Verification items for the finished model (mm, model axes). Coordinates: 2 decimals unless noted, no trailing zeros.
Q1. Cross-section at A-A, the plane y = 1.35. Count the separate pieces of the cut face and the enclosed holes in it, and give its area (3 significant figures).
Q2. Thickness scan on line 1 (X direction, y = 2.6, z = 25) (3 decimals); line 2 (Z direction, x = -38, y = 1.25); line 3 (Z direction, x = 1.5, y = 1.35). Record the ranges inside material, lowest first.
Q3. Depth check by flat-ended pin: P1, Ø5, axis at x = -38.1, z = -66.675, coming from the +Y side (3 decimals); P2, Ø2.5, axis at x = 14.22, z = 83.02, coming from the +Y side. Enter the tip coordinate at first touch or a pass-through.
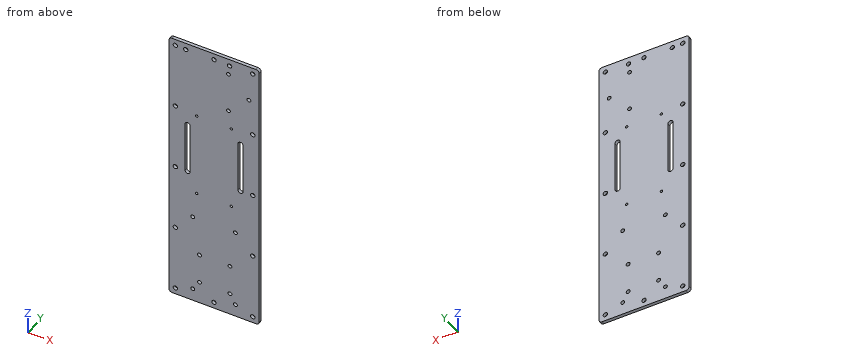
from build123d import *

# Parameters (mm, degrees)
PLATE_THICKNESS_DEPTH      = 3.175
SKETCH3_R                  = 2.159
MOUNTING_HOLES_DEPTH       = 147.635511132
SKETCH4_R                  = 1.905
JETSON_HOLES_W_MOUNT_DEPTH = 147.635511132
SKETCH5_R                  = 1.905
PDB_HOLES_DEPTH            = 147.635511132
SKETCH6_R                  = 1.905
LIDAR_HOLES_DEPTH          = 147.635511132
SKETCH7_R                  = 1.27
PIXHAWK_HOLES_DEPTH        = 147.635511132
BATTERY_HOLES_DEPTH        = 147.635511132
SKETCH9_R                  = 2.159
CUT_EXTRUDE1_DEPTH         = 147.635511132


with BuildPart() as part:
    # Sketch2 → Plate Thickness (new body)
    with BuildSketch(Plane(origin=(0, 0, 0), x_dir=(1, 0, 0), z_dir=(0, 1, 0))):
        with BuildLine():
            Line((-41.275, 139.7), (41.275, 139.7))
            ThreePointArc((41.275, 139.7), (43.52006403, 138.77006403), (44.45, 136.525))
            Line((44.45, 136.525), (44.45, -136.525))
            ThreePointArc((44.45, -136.525), (43.52006403, -138.77006403), (41.275, -139.7))
            Line((41.275, -139.7), (-41.275, -139.7))
            ThreePointArc((-41.275, -139.7), (-43.52006403, -138.77006403), (-44.45, -136.525))
            Line((-44.45, -136.525), (-44.45, 136.525))
            ThreePointArc((-44.45, 136.525), (-43.52006403, 138.77006403), (-41.275, 139.7))
        make_face()
    extrude(amount=PLATE_THICKNESS_DEPTH)

    # Sketch3 → Mounting holes (cut, through all)
    with BuildSketch(Plane(origin=(0, 3.175, 0), x_dir=(1, 0, 0), z_dir=(0, 1, 0))):
        with Locations(Location((-38.1, 133.35, 0), (0, 0, 270))):
            Circle(SKETCH3_R)
        with Locations(Location((-38.1, 66.675, 0), (0, 0, 270))):
            Circle(SKETCH3_R)
        with Locations(Location((-38.1, -66.675, 0), (0, 0, 90))):
            Circle(SKETCH3_R)
        with Locations(Location((-38.1, -133.35, 0), (0, 0, 90))):
            Circle(SKETCH3_R)
        with Locations(Location((38.1, -133.35, 0), (0, 0, 270))):
            Circle(SKETCH3_R)
        with Locations(Location((38.1, -66.675, 0), (0, 0, 270))):
            Circle(SKETCH3_R)
        with Locations(Location((38.1, 66.675, 0), (0, 0, 90))):
            Circle(SKETCH3_R)
        with Locations(Location((38.1, 133.35, 0), (0, 0, 90))):
            Circle(SKETCH3_R)
        with Locations(Location((0, 133.35, 0), (0, 0, 270))):
            Circle(SKETCH3_R)
        with Locations(Location((0, -133.35, 0), (0, 0, 90))):
            Circle(SKETCH3_R)
        with Locations(Location((-38.1, 0, 0), (0, 0, 270))):
            Circle(SKETCH3_R)
        with Locations(Location((38.1, 0, 0), (0, 0, 90))):
            Circle(SKETCH3_R)
    extrude(amount=-MOUNTING_HOLES_DEPTH, mode=Mode.SUBTRACT)

    # Sketch4 → Jetson Holes (w/ mount) (cut, through all)
    with BuildSketch(Plane(origin=(0, 3.175, 0), x_dir=(1, 0, 0), z_dir=(0, 1, 0))):
        with Locations(Location((-21.0058, 127.075242309, 0), (0, 0, 270))):
            Circle(SKETCH4_R)
        with Locations(Location((-21.0058, 48.081242309, 0), (0, 0, 270))):
            Circle(SKETCH4_R)
        with Locations(Location((21.0058, 48.081242309, 0), (0, 0, 90))):
            Circle(SKETCH4_R)
        with Locations(Location((21.0058, 127.075242309, 0), (0, 0, 90))):
            Circle(SKETCH4_R)
    extrude(amount=-JETSON_HOLES_W_MOUNT_DEPTH, mode=Mode.SUBTRACT)

    # Sketch5 → PDB holes (cut, through all)
    with BuildSketch(Plane(origin=(0, 3.175, 0), x_dir=(1, 0, 0), z_dir=(0, 1, 0))):
        with Locations(Location((-14.341868752, 117.235149692, 0), (0, 0, 270))):
            Circle(SKETCH5_R)
        with Locations(Location((15.655531248, 117.235149692, 0), (0, 0, 270))):
            Circle(SKETCH5_R)
        with Locations(Location((15.655531248, 87.237749692, 0), (0, 0, 270))):
            Circle(SKETCH5_R)
        with Locations(Location((-14.341868752, 87.237749692, 0), (0, 0, 270))):
            Circle(SKETCH5_R)
    extrude(amount=-PDB_HOLES_DEPTH, mode=Mode.SUBTRACT)

    # Sketch6 → Lidar Holes (cut, through all)
    with BuildSketch(Plane(origin=(0, 3.175, 0), x_dir=(1, 0, 0), z_dir=(0, 1, 0))):
        with Locations(Location((34.29, -103.082806339, 0), (0, 0, 270))):
            Circle(SKETCH6_R)
        with Locations(Location((14.224, -83.016806339, 0), (0, 0, 270))):
            Circle(SKETCH6_R)
        with Locations(Location((14.224, -123.148806339, 0), (0, 0, 270))):
            Circle(SKETCH6_R)
    extrude(amount=-LIDAR_HOLES_DEPTH, mode=Mode.SUBTRACT)

    # Sketch7 → PixHawk Holes (cut, through all)
    with BuildSketch(Plane(origin=(0, 3.175, 0), x_dir=(1, 0, 0), z_dir=(0, 1, 0))):
        with Locations(Location((-17.145, 20.769931445, 0), (0, 0, 270))):
            Circle(SKETCH7_R)
        with Locations(Location((-17.145, -64.320068555, 0), (0, 0, 270))):
            Circle(SKETCH7_R)
        with Locations(Location((17.145, -64.320068555, 0), (0, 0, 270))):
            Circle(SKETCH7_R)
        with Locations(Location((17.145, 20.769931445, 0), (0, 0, 270))):
            Circle(SKETCH7_R)
    extrude(amount=-PIXHAWK_HOLES_DEPTH, mode=Mode.SUBTRACT)

    # Sketch8 → Battery Holes (cut, through all)
    with BuildSketch(Plane(origin=(0, 3.175, 0), x_dir=(1, 0, 0), z_dir=(0, 1, 0))):
        with BuildLine():
            Line((-23.495, -0.005964701), (-23.495, -50.805964701))
            ThreePointArc((-23.495, -50.805964701), (-26.035, -53.345964701), (-28.575, -50.805964701))
            Line((-28.575, -50.805964701), (-28.575, -0.005964701))
            ThreePointArc((-28.575, -0.005964701), (-26.035, 2.534035299), (-23.495, -0.005964701))
        make_face()
        with BuildLine():
            Line((23.495, -0.005964701), (23.495, -50.805964701))
            ThreePointArc((23.495, -50.805964701), (26.035, -53.345964701), (28.575, -50.805964701))
            Line((28.575, -50.805964701), (28.575, -0.005964701))
            ThreePointArc((28.575, -0.005964701), (26.035, 2.534035299), (23.495, -0.005964701))
        make_face()
    extrude(amount=-BATTERY_HOLES_DEPTH, mode=Mode.SUBTRACT)

    # Sketch9 → Cut-Extrude1 (cut, through all)
    with BuildSketch(Plane(origin=(0, 3.175, 0), x_dir=(1, 0, 0), z_dir=(0, 1, 0))):
        with Locations(Location((-27.868680575, -132.830834732, 0), (0, 0, 270))):
            Circle(SKETCH9_R)
        with Locations(Location((15.311319425, -132.830834732, 0), (0, 0, 270))):
            Circle(SKETCH9_R)
    extrude(amount=-CUT_EXTRUDE1_DEPTH, mode=Mode.SUBTRACT)


solid = part.part
Check values:
1. separate pieces: 1
1. enclosed holes: 31
1. area: 23,900 mm2
2. line 1: x = -44.45 to -28.575, -23.495 to 23.495, 28.575 to 44.45
2. line 2: z = -139.7 to -135.51, -131.19 to -68.83, -64.52 to -2.16, 2.16 to 64.52, 68.83 to 131.19, 135.51 to 139.7
2. line 3: z = -139.7 to -134.9, -131.8 to 131.8, 134.9 to 139.7
3. P1: stops at y = 3.175
3. P2: passes through
